Check sheet for the modelled part. Datum: model origin and axes. Units: mm. Face numbers are marked on the shaded views. A direction names the side the tool comes from. Coordinates: 2 decimals unless noted, no trailing zeros. Loops run counter-clockwise (first coordinate to the right, second up) from the corner with the lowest first, then second, coordinate; pieces in that order, holes last.
```python
from build123d import *

# Parameters (mm, degrees)
SKETCH1_W           = 12.25
SKETCH1_H           = 42.3
BOSS_EXTRUDE1_DEPTH = 7.375
SKETCH2_R           = 1.825
SKETCH2_R_2         = 2.5
CUT_EXTRUDE1_DEPTH  = 24.22129949
CUT_EXTRUDE2_DEPTH  = 24.22129949
SKETCH4_R           = 11.5
CUT_EXTRUDE3_DEPTH  = 5.375
BOSS_EXTRUDE2_START = 0.5
SKETCH5_R           = 4.8
SKETCH5_R_2         = 2.5
BOSS_EXTRUDE2_DEPTH = 0.5
BOSS_EXTRUDE3_START = 4.875
SKETCH6_R           = 3.8
SKETCH6_R_2         = 2.5
BOSS_EXTRUDE3_DEPTH = 4.875
BOSS_EXTRUDE4_REACH = 27.53
CUT_EXTRUDE4_DEPTH  = 26.529896802


with BuildPart() as part:
    # Sketch1 → Boss-Extrude1 (new body)
    with BuildSketch(Plane.XY):
        Rectangle(SKETCH1_W, SKETCH1_H)
    extrude(amount=BOSS_EXTRUDE1_DEPTH)

    # Sketch2 → Cut-Extrude1 (cut, through all)
    with BuildSketch(Plane.XY.offset(7.375)):
        with Locations((-0.475, 15.5)):
            Circle(SKETCH2_R)
        with Locations((-0.475, 0)):
            Circle(SKETCH2_R_2)
    extrude(amount=-CUT_EXTRUDE1_DEPTH, mode=Mode.SUBTRACT)

    # Sketch3 → Cut-Extrude2 (cut, through all)
    with BuildSketch(Plane.XY.offset(7.375)):
        with BuildLine():
            Line((-6.125, -21.15), (-6.125, -16.783974467))
            ThreePointArc((-6.125, -16.783974467), (-4.066466825, -19.092268783), (-1.757457575, -21.15))
            Line((-1.757457575, -21.15), (-6.125, -21.15))
        make_face()
        with BuildLine():
            Line((-6.125, 16.789834467), (-6.125, 21.15))
            Line((-6.125, 21.15), (-1.764842259, 21.15))
            ThreePointArc((-1.764842259, 21.15), (-4.069800152, 19.094796032), (-6.125, 16.789834467))
        make_face()
        with BuildLine():
            Line((6.125, -4.351807973), (6.125, -21.15))
            Line((6.125, -21.15), (1.151863079, -21.15))
            ThreePointArc((1.151863079, -21.15), (2.238128282, -12.336341525), (6.125, -4.351807973))
        make_face()
    extrude(amount=-CUT_EXTRUDE2_DEPTH, mode=Mode.SUBTRACT)

    # Sketch4 → Cut-Extrude3 (cut)
    with BuildSketch(Plane.XY.offset(7.375)):
        with Locations((-0.475, 0)):
            Circle(SKETCH4_R)
    extrude(amount=-CUT_EXTRUDE3_DEPTH, mode=Mode.SUBTRACT)

    # Sketch5 → Boss-Extrude2 (add)
    with BuildSketch(Plane.XY.offset(2).offset(BOSS_EXTRUDE2_START)):
        with Locations((-0.475, 0)):
            Circle(SKETCH5_R)
        with Locations((-0.475, 0)):
            Circle(SKETCH5_R_2, mode=Mode.SUBTRACT)
    extrude(amount=-BOSS_EXTRUDE2_DEPTH)

    # Sketch6 → Boss-Extrude3 (add)
    with BuildSketch(Plane.XY.offset(2.5).offset(BOSS_EXTRUDE3_START)):
        with Locations((-0.475, 0)):
            Circle(SKETCH6_R)
        with Locations((-0.475, 0)):
            Circle(SKETCH6_R_2, mode=Mode.SUBTRACT)
    extrude(amount=-BOSS_EXTRUDE3_DEPTH)

    # Sketch7 → Boss-Extrude4 (add, up to next)
    with BuildSketch(Plane(origin=(-6.125, 0, 0), x_dir=(0, 0, -1), z_dir=(1, 0, 0)), mode=Mode.PRIVATE) as boss_extrude4_sk1:
        with BuildLine():
            Line((-7.375, -13.721160181), (-7.375, -20.698803049))
            ThreePointArc((-7.375, -20.698803049), (-2.25, -17.209981615), (-7.375, -13.721160181))
        make_face()
    boss_extrude4_tool1 = extrude(boss_extrude4_sk1.sketch, amount=BOSS_EXTRUDE4_REACH, mode=Mode.PRIVATE) - part.part
    add(boss_extrude4_tool1.solids().sort_by_distance((-6.125, -17.209982, 5.119864))[0])

    # Sketch8 → Cut-Extrude4 (cut, through all)
    with BuildSketch(Plane(origin=(-6.125, 0, 0), x_dir=(0, 0, -1), z_dir=(1, 0, 0))):
        with BuildLine():
            Line((-9.3, -17.973571615), (-9.3, -16.459481615))
            ThreePointArc((-9.3, -16.459481615), (-7.5, -14.659481615), (-5.7, -16.459481615))
            Line((-5.7, -16.459481615), (-5.7, -17.973571615))
            ThreePointArc((-5.7, -17.973571615), (-7.5, -19.773571615), (-9.3, -17.973571615))
        make_face()
    extrude(amount=CUT_EXTRUDE4_DEPTH, mode=Mode.SUBTRACT)


solid = part.part
```
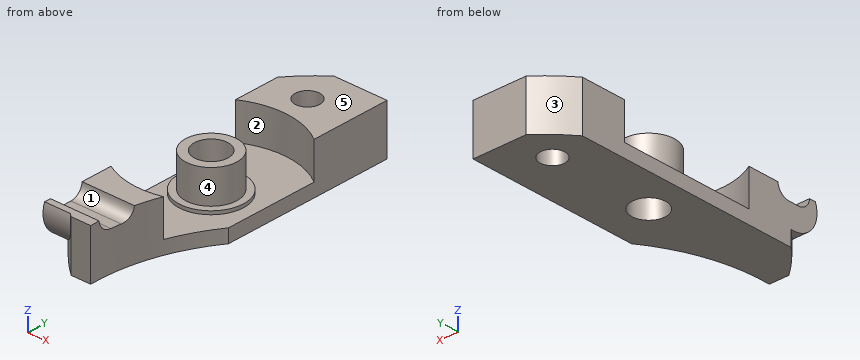
1) Depth check by flat-ended pin: pin 1 (0.8 mm diameter, centred on x = -4, y = -17, fed in from +Z); pin 2 (2 mm diameter, centred on y = -2.5, z = 5, fed in from +X); pin 3 (4 mm diameter, centred on y = -15, z = 6, fed in from +X). Enter the tip coordinate at first touch or a pass-through.
Answer sheet:
pin 1: stops at z = 5.7
pin 2: stops at x = 3.02
pin 3: stops at x = 2.05
2) Section check B-B on z = 4. Enter the section's corners in (x, y) (3 decimals), plus the area to 3 significant figures.
Answer sheet:
outline: (-6.125, -20.382) - (-2.682, -20.382) arc R27 ccw to (-1.757, -21.15) - (1.152, -21.15) arc R27 cw to (2.648, -11.068) arc R11.5 cw to (-6.125, -10.016) - close; (-6.125, 10.016) arc R11.5 cw to (6.125, 9.418) - (6.125, 21.15) - (-1.765, 21.15) arc R27 ccw to (-6.125, 16.79) - close; circle Ø7.6 at (-0.475, 0); hole circle Ø5 at (-0.475, 0); hole circle Ø3.65 at (-0.475, 15.5)
area: 206 mm2
3) Section check D-D on y = -16. Enter the section's corners in (x, z) (3 decimals).
Answer sheet:
outline: (-6.125, 0) - (1.425, 0) - (1.425, 5.76) - (-6.125, 5.76) - close
4) Mould release check, pull along X, two halves, no side actions. Record for the marked faces 1, 2 and 3: +X half, -X half, draft (parallel to the pull), parting line (faces both ways), or undercut.
Answer sheet:
face 1: draft
face 2: undercut
face 3: -X half
5) Section check A-A on y = 0. Enter the section's corners in (x, z) (3 decimals).
Answer sheet:
outline: (-6.125, 0) - (-2.975, 0) - (-2.975, 7.375) - (-4.275, 7.375) - (-4.275, 2.5) - (-5.275, 2.5) - (-5.275, 2) - (-6.125, 2) - close; (2.025, 0) - (6.125, 0) - (6.125, 2) - (4.325, 2) - (4.325, 2.5) - (3.325, 2.5) - (3.325, 7.375) - (2.025, 7.375) - close
6) Set-up check for the marked faces 4 and 5: record each of +Z, -Z, +X, -X, +Y, -Y from which the full face is reachable in a straight line by a thin tool's end or side.
Answer sheet:
face 4: +Z
face 5: +Z, +X, -X, +Y, -Y
7) Section check C-C on y = 15.5. Enter the section's corners in (x, z) (3 decimals).
Answer sheet:
outline: (-6.125, 0) - (-2.3, 0) - (-2.3, 7.375) - (-6.125, 7.375) - close; (1.35, 0) - (6.125, 0) - (6.125, 7.375) - (1.35, 7.375) - close
8) Scan lines: line 1 (Y direction, x = -0.5, z = 1); line 2 (Z direction, x = 5, y = 0); line 3 (Y direction, x = -3.5, z = 5). Record each from-to range of solid material in increasing order.
Answer sheet:
line 1: y = -21.15 to -2.5, 2.5 to 13.68, 17.32 to 21.15
line 2: z = 0 to 2
line 3: y = -20.82 to -11.1, -2.3 to 2.3, 11.1 to 19.65
